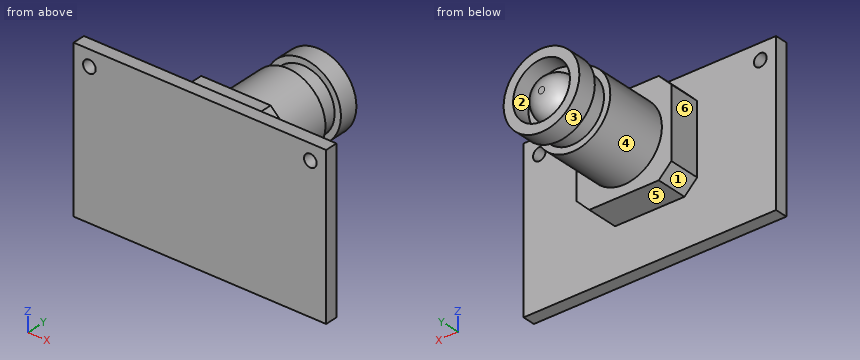
from build123d import *

# Parameters (mm, degrees)
ESQUISSE1_W      = 40
ESQUISSE1_H      = 25
ESQUISSE1_R      = 1
EXTRUSION1_DEPTH = 2
EXTRUSION2_DEPTH = 5
ESQUISSE3_R      = 6
EXTRUSION3_DEPTH = 10
ESQUISSE4_R      = 5
EXTRUSION4_DEPTH = 3
ESQUISSE5_R      = 6
ESQUISSE5_R_2    = 4.5
EXTRUSION5_DEPTH = 3
ESQUISSE6_R      = 3.5
EXTRUSION6_DEPTH = 3
CONG_1_R         = 3


with BuildPart() as part:
    # Esquisse1 → Extrusion1 (new body)
    with BuildSketch(Plane(origin=(0, 0, 0), x_dir=(1, 0, 0), z_dir=(0, 1, 0))):
        with Locations((20, 12.5)):
            Rectangle(ESQUISSE1_W, ESQUISSE1_H)
        with Locations(Location((2.5, 2.5, 0), (0, 0, 270))):
            Circle(ESQUISSE1_R, mode=Mode.SUBTRACT)
        with Locations(Location((37.5, 2.5, 0), (0, 0, 90))):
            Circle(ESQUISSE1_R, mode=Mode.SUBTRACT)
    extrude(amount=EXTRUSION1_DEPTH)

    # Esquisse2 → Extrusion2 (add)
    with BuildSketch(Plane(origin=(0, 2, 0), x_dir=(-1, 0, 0), z_dir=(0, 1, 0))):
        Polygon((-14.5, -17.5), (-25.5, -17.5), (-27.5, -15.5), (-27.5, -4.5), (-25.5, -2.5), (-14.5, -2.5), (-12.5, -4.5), (-12.5, -15.5), align=None)
    extrude(amount=EXTRUSION2_DEPTH)

    # Esquisse3 → Extrusion3 (add)
    with BuildSketch(Plane(origin=(0, 7, 0), x_dir=(1, 0, 0), z_dir=(0, 1, 0))):
        with Locations(Location((20, 10, 0), (0, 0, 90))):
            Circle(ESQUISSE3_R)
    extrude(amount=EXTRUSION3_DEPTH)

    # Esquisse4 → Extrusion4 (add)
    with BuildSketch(Plane(origin=(0, 17, 0), x_dir=(1, 0, 0), z_dir=(0, 1, 0))):
        with Locations(Location((20, 10, 0), (0, 0, 270))):
            Circle(ESQUISSE4_R)
    extrude(amount=EXTRUSION4_DEPTH)

    # Esquisse5 → Extrusion5 (add)
    with BuildSketch(Plane(origin=(0, 20, 0), x_dir=(1, 0, 0), z_dir=(0, 1, 0))):
        with Locations(Location((20, 10, 0), (0, 0, 90))):
            Circle(ESQUISSE5_R)
        with Locations(Location((20, 10, 0), (0, 0, 270))):
            Circle(ESQUISSE5_R_2, mode=Mode.SUBTRACT)
    extrude(amount=EXTRUSION5_DEPTH)

    # Esquisse6 → Extrusion6 (add)
    with BuildSketch(Plane(origin=(0, 20, 0), x_dir=(1, 0, 0), z_dir=(0, 1, 0))):
        with Locations(Location((20, 10, 0), (0, 0, 270))):
            Circle(ESQUISSE6_R)
    extrude(amount=EXTRUSION6_DEPTH)

    # Congé1
    cong_1_edges = [part.edges().sort_by_distance(p)[0] for p in [
        (20, 23, -13.5),
    ]]
    fillet(cong_1_edges, radius=CONG_1_R - 0.0001)  # a hair under: the kernel refuses the full size


solid = part.part
Design review of the part built by this model. Coordinates are the model's own, in mm. Face numbers are marked on the shaded views. A direction names the side the tool comes from. Give positions to 0.01 mm unless a question says otherwise; leave off trailing zeros. Loops run counter-clockwise (first coordinate to the right, second up) from the corner with the lowest first, then second, coordinate; pieces in that order, holes last. Notation, with made-up numbers: M 64.25,52.25 L 100.25,52.25 A16 ccw 100.25,71.25 Z; hole C 63,43.25 d8. An arc over 180 degrees is marked long. One line per question, with ' | ' between items. Start each with the question number.
1. For the marked faces 4, 5 and 6, list the 3-axis set-ups (+Z, -Z, +X, -X, +Y, -Y) from which the entire face can be reached by the end or side of a thin tool; tool diameter is ignored.
2. Add section A-A (x = 2.5). Write out the cut boundary in (y, z), plus the area to 3 significant figures.
3. To check wall thickness, follow L1, parallel to X at y = 0.65, z = -2.5; L2, parallel to Z at x = 37.5, y = 1.4; L3, parallel to X at y = 20.7, z = -10. State the ranges of each line that lie inside material, in increasing order.
4. Add section D-D (y = 7.75). Write out the cut boundary in (x, z).
5. The part is to be moulded in two halves that separate along X. For the marked faces 1, 2 and 3, say which applies: released by +X, released by -X, zero draft, split by the parting line, or undercut.
6. Insertion check: P1, Ø7, axis at x = 18.5, z = -9, coming from the +Y side; P2, Ø10, axis at y = 19.5, z = -16.5, coming from the +X side; P3, Ø2.5, axis at y = 4, z = -11.5, coming from the -X side; P4, Ø3, axis at x = 37.5, z = -2.5, coming from the +Y side. Each pin has a flat end and moves straight along its axis. Give the tip position at first contact, or say it passes through.
7. Add section B-B (x = 13). Write out the cut boundary in (y, z), plus the area to 3 significant figures.
8. Add section C-C (z = -16.5). Write out the cut boundary in (x, y).
Worked out:
1) face 4: +Y | face 5: -Z, +X, -X, +Y | face 6: +Z, -Z, -X, +Y
2) outline: M 0,-25 L 2,-25 L 2,-3.5 L 0,-3.5 Z; M 0,-1.5 L 2,-1.5 L 2,0 L 0,0 Z | area: 46.0 mm²
3) L1: x = 0 to 1.5, 3.5 to 36.5, 38.5 to 40 | L2: z = -25 to -3.5, -1.5 to 0 | L3: x = 14 to 15.5, 16.58 to 23.42, 24.5 to 26
4) outline: C 20,-10 d12
5) face 1: released by -X | face 2: undercut | face 3: split by the parting line
6) P1: stops at y = 23 | P2: stops at x = 25.8 | P3: stops at x = 12.5 | P4: stops at y = 2
7) outline: M 0,-25 L 2,-25 L 2,-16 L 7,-16 L 7,-4 L 2,-4 L 2,0 L 0,0 Z | area: 110 mm²
8) outline: M 0,0 L 40,0 L 40,2 L 26.5,2 L 26.5,7 L 13.5,7 L 13.5,2 L 0,2 Z
